Part print with two shaded views. Sizes in mm from the minimum x, y, z corner. A direction names the side the tool comes from. Round coordinates to 2 decimals unless told otherwise and drop trailing zeros. Write each loop counter-clockwise with the first axis right and the second up, starting at its lowest first coordinate (ties: lowest second). Pieces come first, ordered by that corner, then holes. Notation, with made-up numbers: (54.25, -8) -> (111.25, -8) arc R12 ccw to (111.25, 13) -> close; hole circle Ø11 at (61.5, 60). An arc over 180 degrees is marked (long way). Return JSON: item names as keys, results as strings. Group by question number.
(1) Tool access for the marked faces 3, 4 and 5: list every direction of +Z, -Z, +X, -X, +Y, -Y with a clear straight run to the whole face (end or side of a thin tool).
(2) Drop flat-ended pins along their axis: pin 1 Ø6 at (x, z) = (32, 39.5) entering from +Y; pin 2 Ø3.5 at (x, y) = (12, 42.49) entering from -Z; pin 3 Ø10 at (x, z) = (32.5, 10) entering from -Y; pin 4 Ø5 at (x, y) = (27, 42.49) entering from +Z. Give the stop position or say it passes through.
(3) Saw through at C-C (y = 50). List the corners of the cut face in (x, z).
(4) Saw through at A-A (z = 38.5). List the corners of the cut face in (x, y).
(5) Mould opens along Y. For the marked faces 1 and 2 say: +Y half, -Y half, draft (parallel to the pull), parting line (faces both ways), or undercut.
(6) Drill centre lines: L1, parallel to Y at x = 1.05, z = 38.5; L2, parallel to Y at x = 19.5, z = 21; L3, parallel to X at y = 29, z = 29. Where is each one in solid material? Low to high. Write a range as from..to.
(7) Saw through at B-B (y = 5). List the corners of the cut face in (x, z), plus the area to 3 significant figures.
(8) Saw through at D-D (z = 5). List the corners of the cut face in (x, y).
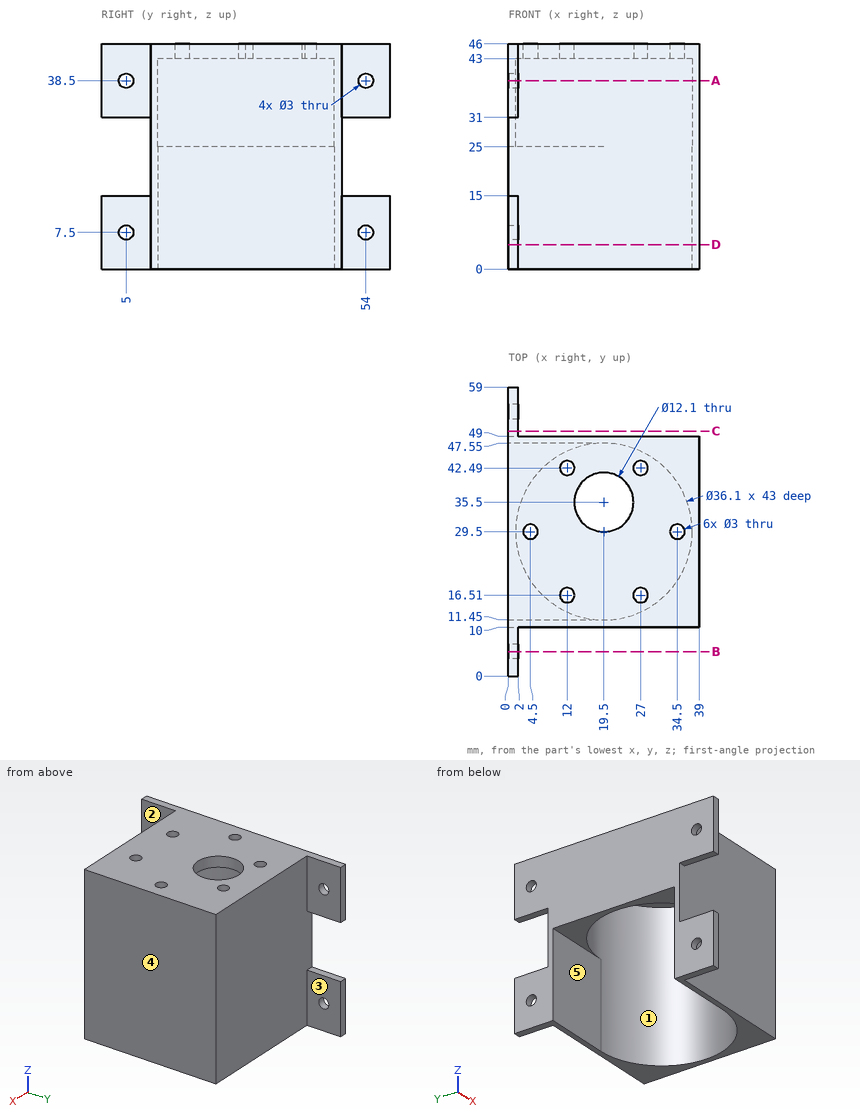
Computed values:
{
 "1": {"face 3": "+Z, -Z, +X, +Y", "face 4": "+Z, -Z, +X, +Y, -Y", "face 5": "-Z, -X"},
 "2": {"pin 1": "y = 49", "pin 2": "z = 43", "pin 3": "y = 10", "pin 4": "z = 46"},
 "3": {"outline": "(0, 0) -> (2, 0) -> (2, 15) -> (0, 15) -> close; (0, 31) -> (2, 31) -> (2, 46) -> (0, 46) -> close"},
 "4": {"outline": "(0, 0) -> (2, 0) -> (2, 3.5) -> (0, 3.5) -> close; (0, 6.5) -> (2, 6.5) -> (2, 10) -> (39, 10) -> (39, 49) -> (2, 49) -> (2, 52.5) -> (0, 52.5) -> close; (0, 55.5) -> (2, 55.5) -> (2, 59) -> (0, 59) -> close; hole circle Ø36.1 at (19.5, 29.5)"},
 "5": {"face 1": "undercut", "face 2": "draft"},
 "6": {"L1": "0..3.5, 6.5..52.5, 55.5..59", "L2": "10..11.45, 47.55..49", "L3": "0..1.46, 37.54..39"},
 "7": {"outline": "(0, 0) -> (2, 0) -> (2, 6) -> (0, 6) -> close; (0, 9) -> (2, 9) -> (2, 15) -> (0, 15) -> close; (0, 31) -> (2, 31) -> (2, 37) -> (0, 37) -> close; (0, 40) -> (2, 40) -> (2, 46) -> (0, 46) -> close", "area": "48.0 mm2"},
 "8": {"outline": "(0, 0) -> (2, 0) -> (2, 10) -> (39, 10) -> (39, 49) -> (2, 49) -> (2, 59) -> (0, 59) -> (0, 47.55) -> (19.5, 47.55) arc R18.05 cw to (19.5, 11.45) -> (0, 11.45) -> close"}
}
